For this review, take the finished solid that the model builds, in its own axes (mm). Coordinates: 2 decimals unless noted, no trailing zeros. Write each loop counter-clockwise with the first axis right and the second up, starting at its lowest first coordinate (ties: lowest second). Pieces come first, ordered by that corner, then holes. Notation, with made-up numbers: M 58.25,3.5 L 81.25,3.5 A24 cw 81.25,14.5 Z; hole C 18,13.5 d7. An arc over 180 degrees is marked long. Return JSON: item names as keys, results as strings.
Autodesk Inventor part; units mm, degrees
ref_plane "YZ Plane" through (0, 0, 0) normal (1, 0, 0) x (0, 1, 0)
ref_plane "XZ Plane" through (0, 0, 0) normal (0, 1, 0) x (-1, 0, 0)
ref_plane "XY Plane" through (0, 0, 0) normal (0, 0, 1) x (1, 0, 0)
sketch "Sketch1" plane through (0, 0, 0) normal (0, 0, 1) x (1, 0, 0)
  line L0 (-100, -100) -> (100, -100)
  line L1 (100, -100) -> (100, 100)
  line L2 (100, 100) -> (-100, 100)
  line L3 (-100, 100) -> (-100, -100)
  line L4 (-100, -100) -> (100, 100) construction
  line L5 (100, -100) -> (-100, 100) construction
  circle A0 centre (60, -60) radius 10
  line L6 (-40, 100) -> (-40, 40)
  line L7 (-40, 40) -> (-100, 40)
  point P0 (0, 0)
  dimension "d154" = 200
  dimension "d155" = 200
  dimension "d157" = 20
  dimension "d158" = 40
  dimension "d159" = 40
  dimension "d161" = 60
extrude "Plate5" add sketch "Sketch1" along normal blind 8
fillet "Corner Round1" radius 30 2 edges at (100, -100, 4) (-100, 100, 4)
properties part number "PNS-071 stretch ring" material "Stainless Steel"
1. We need section A-A (y = -60). State the section outline as (x, z) points, plus the area to 3 significant figures.
Checks:
{"outline": "M -100,0 L 50,0 L 50,8 L -100,8 Z; M 70,0 L 100,0 L 100,8 L 70,8 Z", "area": "1,440 mm2"}
2. We need section B-B (x = 60). State the section outline as (y, z) points, plus the area to 3 significant figures.
Checks:
{"outline": "M -100,0 L -70,0 L -70,8 L -100,8 Z; M -50,0 L 100,0 L 100,8 L -50,8 Z", "area": "1,440 mm2"}
3. Draft analysis for pull direction Y (two halves, no side actions). For faces 1 (the face through (-16, -100, 4)), 2 (the face through (-90.979, 91.445, 4.056)), 3 (the face through (50, -60, 4)), state which applies: +Y half, -Y half, draft (parallel to the pull), parting line (faces both ways), or undercut.
Checks:
{"face 1": "-Y half", "face 2": "+Y half", "face 3": "undercut"}
4. We need section C-C (z = 3.5). State the section outline as (x, y) points, plus the area to 3 significant figures.
Checks:
{"outline": "M -100,-100 L 70,-100 A30 ccw 100,-70 L 100,100 L -70,100 A30 ccw -100,70 Z; hole C 60,-60 d20", "area": "39,300 mm2"}
5. Wall thickness on L1, parallel to X at y = -60.5, z = 5.5; L2, parallel to Y at x = 60, z = 3.25; L3, parallel to Y at x = 58.5, z = 5: over which ranges is each line inside the solid? List them lowest first. Write a range as from..to.
Checks:
{"L1": "-100..50.01, 69.99..100", "L2": "-100..-70, -50..100", "L3": "-100..-69.89, -50.11..100"}
